Autodesk Inventor part; units mm, degrees
ref_plane "Work Plane2" through (-21.474, 0, -18.2189) normal (-1, 0, 0) x (0, 0, 1)
ref_plane "YZ Plane" through (0, 0, 0) normal (1, 0, 0) x (0, 1, 0)
ref_plane "XZ Plane" through (0, 0, 0) normal (0, 1, 0) x (-1, 0, 0)
sketch "Sketch1" plane through (0, 0, 0) normal (0, 1, 0) x (-1, 0, 0)
  line L0 (71.974, 9.2811) -> (-6.026, 9.2811)
  line L1 (-6.026, 9.2811) -> (-6.026, -18.2189)
  line L2 (-6.026, -18.2189) -> (71.974, -18.2189)
  line L3 (71.974, -18.2189) -> (71.974, 9.2811)
  point P0 (0, 0)
  dimension "d0" = 27.5
  dimension "d1" = 78
extrude "Extrusion1" add sketch "Sketch1" along normal blind 9
sketch "Sketch2" plane through (0, 9, 0) normal (0, 1, 0) x (1, 0, 0)
  line L0 (6.026, 18.2189) -> (-71.974, 18.2189)
  line L1 (-71.974, -9.2811) -> (6.026, -9.2811)
  line L2 (6.026, 18.2189) -> (-19.474, 18.2189)
  line L3 (-19.474, 18.2189) -> (-19.474, -9.2811)
  line L4 (-19.474, -9.2811) -> (6.026, -9.2811)
  line L5 (6.026, -9.2811) -> (6.026, 18.2189)
  point P0 (0, 0)
  point P1 (6.026, -9.2811)
  point P2 (-19.474, 18.2189)
  dimension "d4" = 25.5
extrude "Extrusion2" cut sketch "Sketch2" against normal blind 7
sketch "Sketch3" plane through (0, 2, 0) normal (0, 1, 0) x (1, 0, 0)
  point P0 (0, 0)
sketch "Sketch4" plane through (0, 2, 0) normal (0, 1, 0) x (1, 0, 0)
  line L0 (-19.474, -9.2811) -> (-19.474, 18.2189)
  line L1 (6.026, -9.2811) -> (6.026, 18.2189)
  line L2 (-19.474, 18.2189) -> (6.026, 18.2189)
  line L3 (6.026, 18.2189) -> (6.026, 16.7189)
  line L4 (6.026, 16.7189) -> (-19.474, 16.7189)
  line L5 (-19.474, 16.7189) -> (-19.474, 18.2189)
  point P0 (0, 0)
  point P1 (6.026, 18.2189)
  point P2 (-19.474, 16.7189)
  dimension "d7" = 1.5
extrude "Extrusion3" add sketch "Sketch4" along normal blind 7
sketch "Sketch5" plane through (-71.974, 0, 9.2811) normal (0, 0, 1) x (1, 0, 0)
  line L0 (0, 9) -> (52.5, 9)
  line L1 (50.5, 9) -> (50.5, 0)
  line L2 (0, 0) -> (78, 0)
  line L3 (52.5, 2) -> (52.5, 9)
  line L4 (50.5, 7) -> (0, 7)
  line L5 (52.5, 2) -> (52.5, 9)
  line L6 (0, 9) -> (52.5, 9)
  line L7 (0, 0) -> (0, 9)
  line L8 (0, 0) -> (78, 0)
  line L9 (78, 0) -> (78, 2)
  line L10 (78, 2) -> (52.5, 2)
  point P0 (71.974, 0)
  point P1 (0, 7)
  dimension "d10" = 2
  dimension "d11" = 2
extrude "Extrusion4" cut sketch "Sketch5" against normal blind 44 contours L4 L1 L2 L7
sketch "Sketch8" plane through (-71.974, 7, 9.2811) normal (0, -1, 0) x (1, 0, 0)
  line L0 (50.5, -21.9505) -> (25.5, -21.9505)
  line L1 (25.5, -21.9505) -> (25.5, -4.7505)
  line L2 (25.5, -4.7505) -> (50.5, -4.7505)
  line L3 (50.5, -4.7505) -> (50.5, -21.9505)
  line L4 (50.5, 0) -> (50.5, -27.5)
  point P0 (71.974, -9.2811)
  dimension "d20" = 17.2
  dimension "d21" = 25
  dimension "d22" = 0
extrude "Extrusion6" cut sketch "Sketch8" against normal blind 2
ref_plane "Work Plane2" through (-21.474, 0, -18.2189) normal (-1, 0, 0) x (0, 0, 1)
split "Split2" plane through (-21.474, 0, -18.2189) removes the side toward (1, 0, 0)
sketch "Sketch10" plane through (0, 9, 0) normal (0, 1, 0) x (1, 0, 0)
  line L0 (-71.974, 18.2189) -> (6.026, 18.2189)
  line L1 (6.026, 18.2189) -> (6.026, -9.2811)
  line L2 (6.026, -9.2811) -> (-71.974, -9.2811)
  line L3 (-71.974, -9.2811) -> (-71.974, 18.2189)
  line L4 (-21.474, 12.6694) -> (-46.474, 12.6694)
  line L5 (-21.474, 12.6694) -> (-21.474, -9.2811)
  line L6 (-21.474, -9.2811) -> (-21.474, -4.5306)
  line L7 (-21.474, -4.5306) -> (-46.474, -4.5306)
  line L8 (-46.474, -4.5306) -> (-46.474, 12.6694)
  line L9 (-46.474, 12.6694) -> (-21.474, 12.6694)
  line L10 (-21.474, 12.6694) -> (-21.474, 18.2189)
  line L11 (-21.474, 18.2189) -> (-71.974, 18.2189)
  line L12 (-71.974, 18.2189) -> (-71.974, -9.2811)
  line L13 (-71.974, -9.2811) -> (-21.474, -9.2811)
  point P0 (0, 0)
  dimension "d32" = 78
  dimension "d33" = 27.5
extrude "Extrusion7" add sketch "Sketch10" against normal blind 2 contours L0 L1 L2 L5 L10
sketch "Sketch11" plane through (-71.974, 7, 9.2811) normal (0, 0, 1) x (1, 0, 0)
  line L0 (0, 2) -> (78, 2)
  line L1 (0, 0) -> (0, 2)
  line L2 (78, 0) -> (0, 0)
  line L3 (78, 2) -> (78, 0)
  point P0 (71.974, -7)
extrude "Extrusion8" add sketch "Sketch11" along normal blind 2
sketch "Sketch12" plane through (-71.974, 7, -18.2189) normal (0, -1, 0) x (1, 0, 0)
  line L0 (0, 0) -> (0, 29.5)
  line L1 (78, 0) -> (0, 0)
  line L2 (78, 0) -> (78, 29.5)
  line L3 (0, 29.5) -> (78, 29.5)
  line L4 (50.5, 22.7495) -> (50.5, 5.5495)
  line L5 (50.5, 5.5495) -> (25.5, 5.5495)
  line L6 (25.5, 5.5495) -> (25.5, 22.7495)
  line L7 (25.5, 22.7495) -> (50.5, 22.7495)
  line L8 (78, 0) -> (0, 0)
  line L9 (50.5, 0) -> (25.5, 0)
  line L10 (25.5, 0) -> (25.5, 29.5)
  line L11 (25.5, 29.5) -> (50.5, 29.5)
  line L12 (50.5, 29.5) -> (50.5, 0)
  point P0 (71.974, 18.2189)
  point P1 (50.5, 0)
  point P2 (25.5, 0)
extrude "Extrusion9" cut sketch "Sketch12" against normal blind 1 contours L10 L5 L12 L1 | L3 L12 L7 L10
properties part number "pokrywka"
The listing builds one solid part. Answer for the finished solid, in the listing's coordinates (mm). A direction names the side the tool comes from. Coordinates: 2 decimals unless noted, no trailing zeros. Loops run counter-clockwise (first coordinate to the right, second up) from the corner with the lowest first, then second, coordinate; pieces in that order, holes last.
1) Find the intervals of material crossed by L1, parallel to X at y = 7.5, z = 6.75; L2, parallel to Z at x = -30.5, y = 8.3; L3, parallel to Y at x = -41.5, z = -14.5, in increasing order.
2) Find section A-A on z = 0.75. Write down the section's boundary in (x, y).
3) Find section B-B on y = 7.4. Write down the section's boundary in (x, z).
4) A tool of negligible diameter and unlimited length cuts with its end or side. For faces 4 (the face through (-34, 8, -15)), 5 (the face through (-46.474, 8, -4)), 6 (the face through (-59, 7, -4)), from which of +Z, -Z, +X, -X, +Y, -Y can it reach the whole face along a straight path? Write none if from no direction.
5) A flat-ended cylindrical pin translates along its axis: pin 1 Ø2 at (x, z) = (-39.5, 8.5) entering from -Y. Find the tip coordinate at first contact, or state that the pin passes through.
6) Determine the mould class of faces 1 (the face through (-8, 7, -4)), 2 (the face through (-71.974, 8, -4)), 3 (the face through (-21.474, 8, -4)) for opening direction X: pulls with the +X half, pulls with the -X half, needs draft (parallel to the pull), parting line crosses it, or undercut.
7) Find section C-C on z = 9.5. Write down the section's boundary in (x, y).
Values:
1. L1: x = -71.97 to -46.47, -21.47 to 6.03
1. L2: z = -18.22 to -12.67, 4.53 to 11.28
1. L3: y = 8 to 9
2. outline: (-71.97, 7) - (-46.47, 7) - (-46.47, 9) - (-71.97, 9) - close; (-21.47, 7) - (6.03, 7) - (6.03, 9) - (-21.47, 9) - close
3. outline: (-71.97, -18.22) - (-46.47, -18.22) - (-46.47, 11.28) - (-71.97, 11.28) - close; (-21.47, -18.22) - (6.03, -18.22) - (6.03, 11.28) - (-21.47, 11.28) - close
4. face 4: +Z, -Z, -Y
4. face 5: -Y
4. face 6: +Z, -Z, +X, -X, -Y
5. pin 1: stops at y = 8
6. face 1: needs draft
6. face 2: pulls with the -X half
6. face 3: undercut
7. outline: (-71.97, 7) - (-46.47, 7) - (-46.47, 8) - (-21.47, 8) - (-21.47, 7) - (6.03, 7) - (6.03, 9) - (-71.97, 9) - close
